Check sheet for the modelled part. Datum: model origin and axes. Units: mm. A direction names the side the tool comes from. Coordinates: 2 decimals unless noted, no trailing zeros. Write each loop counter-clockwise with the first axis right and the second up, starting at its lowest first coordinate (ties: lowest second). Pieces come first, ordered by that corner, then holes. Notation, with made-up numbers: M -9.5,25 L 38.5,25 A12 cw 38.5,46 Z; hole C 39.25,34.5 d1. An arc over 180 degrees is marked long. Answer as CSV lines item,"result". Start each with the question number.
1) Go/stop test with flat-tipped pins: pin 1 Ø4 at (x, z) = (-0.5, -9) entering from +Y; pin 2 Ø1.6 at (x, z) = (-5, -12.5) entering from +Y; pin 3 Ø1.5 at (y, z) = (16, 7.5) entering from -X. Record where each tip stops, or that it passes through.
2) Section check D-D (z = -5.25). Record the cut outline in (x, y).
3) Access from +Z, -Z, +X, -X, +Y, -Y to the whole of each face (thin tool, end or side, straight path). Record for faces 5 (the flat face through (0, -10, -8)), 6 (the cylindrical face through (25.865, -10.724, 2.465)), 7 (the flat face through (0, -19.75, -13)).
4) Section check A-A (x = -13). Record the cut outline in (y, z), and give its area (3 significant figures).
5) Material ranges on L1, parallel to Y at x = 0, z = 1.9; L2, parallel to Y at x = 0, z = 3.1; L3, parallel to Z at x = 17.5, y = -7, recorded low to high. Write a range as [from, to].
6) Draft check along X on faces 1 (the flat face through (0, 10, -8)), 2 (the flat face through (8.866, -4.735, 1.479)), 3 (the flat face through (-19.75, 0, -13)), 4 (the flat face through (-25, 13, 5)). Enter one of: +X half, -X half, draft (parallel to the pull), parting line (faces both ways), or undercut.
7) Section check C-C (y = 16.5). Record the cut outline in (x, z), and give its area (3 significant figures).
from build123d import *

# Parameters (mm, degrees)
SKETCH2_R             = 30
SKETCH2_R_2           = 28
BOSS_EXTRUDE1_DEPTH   = 5
SKETCH2_R_3           = 38
SKETCH2_R_4           = 36.5
BOSS_EXTRUDE1_2_DEPTH = 5
SKETCH5_R             = 38
BOSS_EXTRUDE2_DEPTH   = 4
BOSS_EXTRUDE3_DEPTH   = 3
CUT_EXTRUDE1_DEPTH    = 1.5
SKETCH10_R            = 38
SKETCH10_R_2          = 36.5
BOSS_EXTRUDE4_DEPTH   = 8
SKETCH11_W            = 20
SKETCH11_H            = 20
BOSS_EXTRUDE5_DEPTH   = 8
SKETCH12_W            = 39.5
SKETCH12_H            = 39.5
BOSS_EXTRUDE6_DEPTH   = 2


with BuildPart() as part:
    # Sketch2 → Boss-Extrude1 (new body)
    with BuildSketch(Plane.XY):
        Circle(SKETCH2_R)
        Circle(SKETCH2_R_2, mode=Mode.SUBTRACT)
    extrude(amount=BOSS_EXTRUDE1_DEPTH)



with BuildPart() as body_2:
    # Sketch2 → Boss-Extrude1 2 (new body)
    with BuildSketch(Plane.XY):
        Circle(SKETCH2_R_3)
        Circle(SKETCH2_R_4, mode=Mode.SUBTRACT)
    extrude(amount=BOSS_EXTRUDE1_2_DEPTH)


with BuildPart() as part_1:
    add(part.part)

    add(body_2.part)  # Boss-Extrude2 merges body 2
    # Sketch5 → Boss-Extrude2 (add)
    with BuildSketch(Plane(origin=(0, 0, 0), x_dir=(-1, 0, 0), z_dir=(0, 0, -1))):
        Circle(SKETCH5_R)
    extrude(amount=BOSS_EXTRUDE2_DEPTH)

    # Sketch6 → Boss-Extrude3 (add)
    with BuildSketch(Plane.XY):
        with BuildLine():
            Line((0.868619612, 5.441102827), (16.642915533, 4.048692183))
            ThreePointArc((16.642915533, 4.048692183), (20.59, 0), (16.642915533, -4.048692183))
            Line((16.642915533, -4.048692183), (0.868619612, -5.441102827))
            ThreePointArc((0.868619612, -5.441102827), (-5.51, 0), (0.868619612, 5.441102827))
        make_face()
        with BuildLine():
            Line((0.614870513, 3.455724852), (16.54, 2.05))
            ThreePointArc((16.54, 2.05), (18.59, 0), (16.54, -2.05))
            Line((16.54, -2.05), (0.614870513, -3.455724852))
            ThreePointArc((0.614870513, -3.455724852), (-3.51, 0), (0.614870513, 3.455724852))
        make_face(mode=Mode.SUBTRACT)
    extrude(amount=BOSS_EXTRUDE3_DEPTH)

    # Sketch9 → Cut-Extrude1 (cut)
    with BuildSketch(Plane.XY):
        with BuildLine():
            Line((0.614870513, 3.455724852), (16.54, 2.05))
            ThreePointArc((16.54, 2.05), (18.59, 0), (16.54, -2.05))
            Line((16.54, -2.05), (0.614870513, -3.455724852))
            ThreePointArc((0.614870513, -3.455724852), (-3.51, 0), (0.614870513, 3.455724852))
        make_face()
    extrude(amount=-CUT_EXTRUDE1_DEPTH, mode=Mode.SUBTRACT)

    # Sketch10 → Boss-Extrude4 (add)
    with BuildSketch(Plane.XY.offset(5)):
        Circle(SKETCH10_R)
        Circle(SKETCH10_R_2, mode=Mode.SUBTRACT)
    extrude(amount=BOSS_EXTRUDE4_DEPTH)

    # Sketch11 → Boss-Extrude5 (add)
    with BuildSketch(Plane(origin=(0, 0, -4), x_dir=(-1, 0, 0), z_dir=(0, 0, -1))):
        Rectangle(SKETCH11_W, SKETCH11_H)
    extrude(amount=BOSS_EXTRUDE5_DEPTH)

    # Sketch12 → Boss-Extrude6 (add)
    with BuildSketch(Plane(origin=(0, 0, -12), x_dir=(-1, 0, 0), z_dir=(0, 0, -1))):
        Rectangle(SKETCH12_W, SKETCH12_H)
    extrude(amount=BOSS_EXTRUDE6_DEPTH)


solid = part_1.part
Results found:
1,pin 1,"stops at y = 10"
1,pin 2,"stops at y = 19.75"
1,pin 3,"stops at x = -34.81"
2,outline,"M -10,-10 L 10,-10 L 10,10 L -10,10 Z"
3,face 5,"+X, -X, -Y"
3,face 6,"+Z"
3,face 7,"-Z, +X, -X, -Y"
4,outline,"M -35.71,-4 L 35.71,-4 L 35.71,13 L 34.11,13 L 34.11,0 L 27.04,0 L 27.04,5 L 24.8,5 L 24.8,0 L -24.8,0 L -24.8,5 L -27.04,5 L -27.04,0 L -34.11,0 L -34.11,13 L -35.71,13 Z; M -19.75,-14 L 19.75,-14 L 19.75,-12 L -19.75,-12 Z"
4,area,"429 mm2"
5,L1,"y = [-38, -36.5], [-30, -28], [-5.51, -3.51], [3.51, 5.51], [28, 30], [36.5, 38]"
5,L2,"y = [-38, -36.5], [-30, -28], [28, 30], [36.5, 38]"
5,L3,"z = [-14, -12], [-4, 0]"
6,face 1,"draft"
6,face 2,"undercut"
6,face 3,"-X half"
6,face 4,"undercut"
7,outline,"M -34.23,-4 L 34.23,-4 L 34.23,13 L 32.56,13 L 32.56,0 L 25.05,0 L 25.05,5 L 22.62,5 L 22.62,0 L -22.62,0 L -22.62,5 L -25.05,5 L -25.05,0 L -32.56,0 L -32.56,13 L -34.23,13 Z; M -19.75,-14 L 19.75,-14 L 19.75,-12 L -19.75,-12 Z"
7,area,"421 mm2"
